The listing builds one solid part. Answer for the finished solid, in the listing's coordinates (mm). Face numbers are marked on the shaded views. A direction names the side the tool comes from. Round coordinates to 2 decimals unless told otherwise and drop trailing zeros. Order: outer loops, then holes, each group sorted by start corner. A loop starts at its lowest first (then second) coordinate and runs counter-clockwise, first axis right, second up. Notation, with made-up numbers: (23, 68) -> (56, 68) arc R17 ccw to (56, 83) -> close; hole circle Ø1 at (85.25, 85.25). An arc over 180 degrees is marked (long way). Answer in a Markdown table with one row per item. Add a question column.
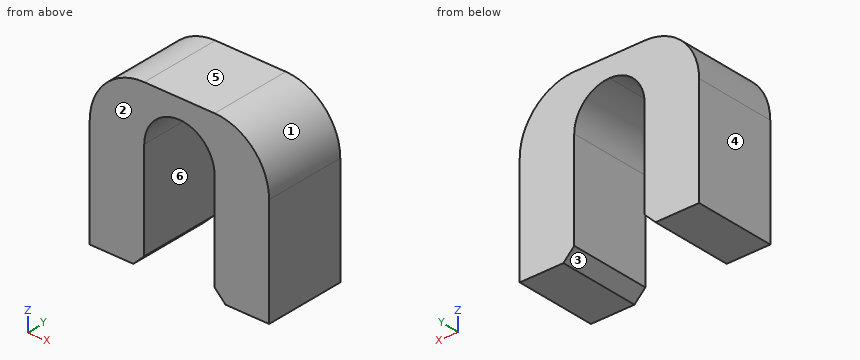
```python
from build123d import *

# Parameters (mm, degrees)
F1_DEPTH = 9.525
F2_R     = 6.35
F3_SIZE  = 1.27


with BuildPart() as f1:
    # F0 (on Front) → F1 (new body)
    with BuildSketch(Plane.XZ):
        with BuildLine():
            Line((-4.1, -12.7), (-4.1, 0))
            ThreePointArc((-4.1, 0), (-2.899138, 2.899138), (0, 4.1))
            Line((0, 4.1), (0, 6.35))
            Line((0, 6.35), (-10.45, 6.35))
            Line((-10.45, 6.35), (-10.45, -12.7))
            Line((-10.45, -12.7), (-4.1, -12.7))
        make_face()
        with BuildLine():
            Line((0, 6.35), (0, 4.1))
            ThreePointArc((0, 4.1), (2.899138, 2.899138), (4.1, 0))
            Line((4.1, 0), (4.1, -12.7))
            Line((4.1, -12.7), (10.45, -12.7))
            Line((10.45, -12.7), (10.45, 6.35))
            Line((10.45, 6.35), (0, 6.35))
        make_face()
    extrude(amount=F1_DEPTH)

    # F2
    f2_edges = [f1.edges().sort_by_distance(p)[0] for p in [
        (-10.45, -4.7625, 6.35),
        (10.45, -4.7625, 6.35),
    ]]
    fillet(f2_edges, radius=F2_R)

    # F3
    f3_edges = [f1.edges().sort_by_distance(p)[0] for p in [
        (-4.1, -4.7625, -12.7),
        (4.1, -4.7625, -12.7),
    ]]
    chamfer(f3_edges, length=F3_SIZE)


solid = f1.part
```
1. The part is cut by section D-D (z = 2.5). Give the vertices of the cut face in (x, y) (3 decimals).
2. The mould has two halves that part along X. Classify the marked faces 1, 2, 3 and 4: released by +X, released by -X, zero draft, split by the parting line, or undercut.
3. The part is cut by section A-A (z = -6). Give the vertices of the cut face in (x, y) (3 decimals).
4. The part is cut by section B-B (y = -6.5). Give the vertices of the cut face in (x, z), then the cut area to 3 significant figures.
5. The part is cut by section C-C (x = 6). Give the vertices of the cut face in (y, z) (3 decimals), then the cut area to 3 significant figures.
6. Straight lines are drawn through the part: line 1 along X through (y, z) = (-4, -6.5); line 2 along X through (y, z) = (-6.75, 5.5). For each, find the intervals that lie inside material, in ascending order.
7. For the marked faces 5 and 6, determine the directions among +Z, -Z, +X, -X, +Y, -Y from which every point of the face is accessible in a straight line to the end or side of a thin tool.
Report:
| question | item | result |
|---|---|---|
| 1 | outline | (-9.937, -9.525) -> (-3.25, -9.525) -> (-3.25, 0) -> (-9.937, 0) -> close; (3.25, -9.525) -> (9.937, -9.525) -> (9.937, 0) -> (3.25, 0) -> close |
| 2 | face 1 | released by +X |
| 2 | face 2 | zero draft |
| 2 | face 3 | undercut |
| 2 | face 4 | released by -X |
| 3 | outline | (-10.45, -9.525) -> (-4.1, -9.525) -> (-4.1, 0) -> (-10.45, 0) -> close; (4.1, -9.525) -> (10.45, -9.525) -> (10.45, 0) -> (4.1, 0) -> close |
| 4 | outline | (-10.45, -12.7) -> (-5.37, -12.7) -> (-4.1, -11.43) -> (-4.1, 0) arc R4.1 cw to (0, 4.1) arc R4.1 cw to (4.1, 0) -> (4.1, -11.43) -> (5.37, -12.7) -> (10.45, -12.7) -> (10.45, 0) arc R6.35 ccw to (4.1, 6.35) -> (-4.1, 6.35) arc R6.35 ccw to (-10.45, 0) -> close |
| 4 | area | 249 mm^2 |
| 5 | outline | (-9.525, -12.7) -> (0, -12.7) -> (0, 6.059) -> (-9.525, 6.059) -> close |
| 5 | area | 179 mm^2 |
| 6 | line 1 | x = -10.45 to -4.1, 4.1 to 10.45 |
| 6 | line 2 | x = -7.27 to 7.27 |
| 7 | face 5 | +Z, +X, -X, +Y, -Y |
| 7 | face 6 | -Z, +Y, -Y |
